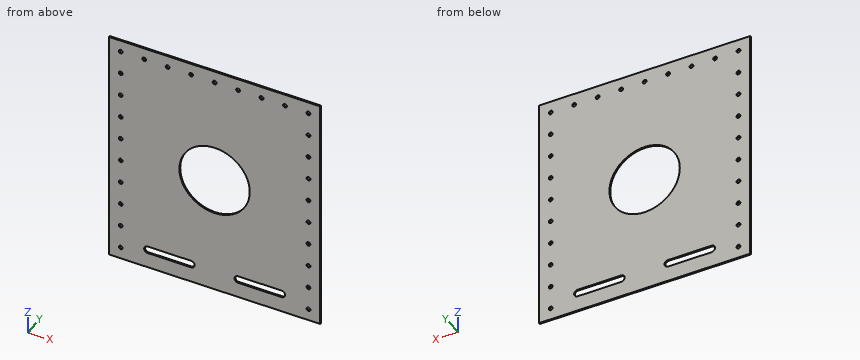
Autodesk Inventor part; units mm, degrees
ref_plane "YZ Plane" through (0, 0, 0) normal (1, 0, 0) x (0, 1, 0)
ref_plane "XZ Plane" through (0, 0, 0) normal (0, 1, 0) x (-1, 0, 0)
ref_plane "XY Plane" through (0, 0, 0) normal (0, 0, 1) x (1, 0, 0)
sketch "Sketch1" plane through (0, 0, 0) normal (0, 1, 0) x (-1, 0, 0)
  line L0 (-114.3, 127) -> (114.3, 127)
  line L1 (114.3, 127) -> (114.3, -127)
  line L2 (114.3, -127) -> (-114.3, -127)
  line L3 (-114.3, -127) -> (-114.3, 127)
  line L4 (-114.3, 127) -> (114.3, -127) construction
  line L5 (114.3, 127) -> (-114.3, -127) construction
  circle A0 centre (101.6, 114.3) radius 2.0701
  circle A1 centre (101.6, 88.9) radius 2.0701
  circle A2 centre (101.6, 63.5) radius 2.0701
  circle A3 centre (101.6, 38.1) radius 2.0701
  circle A4 centre (101.6, 12.7) radius 2.0701
  circle A5 centre (101.6, -12.7) radius 2.0701
  circle A6 centre (101.6, -38.1) radius 2.0701
  circle A7 centre (101.6, -63.5) radius 2.0701
  circle A8 centre (101.6, -88.9) radius 2.0701
  circle A9 centre (101.6, -114.3) radius 2.0701
  circle A10 centre (76.2, 114.3) radius 2.0701
  circle A11 centre (50.8, 114.3) radius 2.0701
  circle A12 centre (25.4, 114.3) radius 2.0701
  circle A13 centre (0, 114.3) radius 2.0701
  circle A14 centre (-25.4, 114.3) radius 2.0701
  circle A15 centre (-50.8, 114.3) radius 2.0701
  circle A16 centre (-76.2, 114.3) radius 2.0701
  circle A17 centre (-101.6, 114.3) radius 2.0701
  circle A18 centre (0, 0) radius 38.1
  circle A19 centre (-101.6, 88.9) radius 2.0701
  circle A20 centre (-101.6, 63.5) radius 2.0701
  circle A21 centre (-101.6, 38.1) radius 2.0701
  circle A22 centre (-101.6, 12.7) radius 2.0701
  circle A23 centre (-101.6, -12.7) radius 2.0701
  circle A24 centre (-101.6, -38.1) radius 2.0701
  circle A25 centre (-101.6, -63.5) radius 2.0701
  circle A26 centre (-101.6, -88.9) radius 2.0701
  circle A27 centre (-101.6, -114.3) radius 2.0701
  dimension "d0" = 228.6
  dimension "d1" = 254
  dimension "d4" = 4.1402
  dimension "d5" = 12.7
  dimension "d6" = 12.7
  dimension "d9" = 25.4
  dimension "d16" = 25.4
  dimension "d28" = 76.2
  dimension "d31" = 25.4
extrude "Extrusion1" add sketch "Sketch1" along normal blind 1.5875
sketch "Sketch2" plane through (0, 1.5875, 0) normal (0, 1, 0) x (1, 0, 0)
  line L0 (72.39, 106.68) -> (25.4, 106.68) construction
  line L1 (72.39, 110.49) -> (25.4, 110.49)
  line L2 (25.4, 102.87) -> (72.39, 102.87)
  arc A0 (72.39, 102.87) -> (72.39, 110.49) centre (72.39, 106.68) ccw
  arc A1 (25.4, 110.49) -> (25.4, 102.87) centre (25.4, 106.68) ccw
  line L3 (114.3, 127) -> (-114.3, 127)
  line L4 (114.3, -127) -> (114.3, 127)
  line L5 (-25.4, 106.68) -> (-72.39, 106.68) construction
  line L6 (-25.4, 110.49) -> (-72.39, 110.49)
  line L7 (-72.39, 102.87) -> (-25.4, 102.87)
  arc A2 (-25.4, 102.87) -> (-25.4, 110.49) centre (-25.4, 106.68) ccw
  arc A3 (-72.39, 110.49) -> (-72.39, 102.87) centre (-72.39, 106.68) ccw
  line L8 (-114.3, 127) -> (-114.3, -127)
  point P0 (0, 0)
  point P1 (48.895, 106.68)
  point P2 (-48.895, 106.68)
  dimension "d36" = 46.99
  dimension "d37" = 7.62
  dimension "d38" = 20.32
  dimension "d39" = 41.91
  dimension "d40" = 46.99
  dimension "d41" = 7.62
  dimension "d42" = 20.32
  dimension "d43" = 41.91
extrude "Extrusion2" cut sketch "Sketch2" against normal blind 25.4
properties part number "ArmPlate" material "Aluminum 6061"
Design review of the part built by this model. Coordinates are the model's own, in mm. Give positions to 0.01 mm unless a question says otherwise; leave off trailing zeros. Write each loop counter-clockwise with the first axis right and the second up, starting at its lowest first coordinate (ties: lowest second). Pieces come first, ordered by that corner, then holes. Notation, with made-up numbers: M 84.25,14.5 L 112.25,14.5 A23 cw 112.25,27.5 Z; hole C 82.25,40 d10. An arc over 180 degrees is marked long. Answer as a JSON object with one key per item and string values. Group by question number.
1) Clearance check with a flat-ended pin moving along its axis: pin 1 Ø3.5 at (x, z) = (-101.6, -63.5) entering from +Y. State where the tip first meets the part, or that it passes through.
2) We need section D-D (x = 32). Give the boundary of the cut face in (y, z).
3) We need section A-A (z = -106.68). Give the boundary of the cut face in (x, y).
4) We need section C-C (z = 0). Give the boundary of the cut face in (x, y).
5) For line 1 along Z through (x, y) = (-70.5, 1); line 2 along X through (y, z) = (1.15, -14); line 3 along Z through (x, y) = (-25.4, 0.5), list the stretches that pass through material, from the lowest coordinate up.
6) We need section B-B (x = -66.5). Give the boundary of the cut face in (y, z), and give its area (3 significant figures).
Answer key:
{
 "1": {"pin 1": "passes through"},
 "2": {"outline": "M 0,-127 L 1.59,-127 L 1.59,-110.49 L 0,-110.49 Z; M 0,-102.87 L 1.59,-102.87 L 1.59,-20.68 L 0,-20.68 Z; M 0,20.68 L 1.59,20.68 L 1.59,127 L 0,127 Z"},
 "3": {"outline": "M -114.3,0 L -76.2,0 L -76.2,1.59 L -114.3,1.59 Z; M -21.59,0 L 21.59,0 L 21.59,1.59 L -21.59,1.59 Z; M 76.2,0 L 114.3,0 L 114.3,1.59 L 76.2,1.59 Z"},
 "4": {"outline": "M -114.3,0 L -38.1,0 L -38.1,1.59 L -114.3,1.59 Z; M 38.1,0 L 114.3,0 L 114.3,1.59 L 38.1,1.59 Z"},
 "5": {"line 1": "z = -127 to -110.49, -102.87 to 127", "line 2": "x = -114.3 to -103.21, -99.99 to -35.43, 35.43 to 99.99, 103.21 to 114.3", "line 3": "z = -127 to -110.49, -102.87 to -28.4, 28.4 to 112.23, 116.37 to 127"},
 "6": {"outline": "M 0,-127 L 1.59,-127 L 1.59,-110.49 L 0,-110.49 Z; M 0,-102.87 L 1.59,-102.87 L 1.59,127 L 0,127 Z", "area": "391 mm²"}
}
